Drawing for the job (mm, zero at the part's lowest x, y, z). Give positions to 0.01 mm unless a question says otherwise; leave off trailing zeros. Loops run counter-clockwise (first coordinate to the right, second up) from the corner with the lowest first, then second, coordinate; pieces in that order, holes last. Notation, with made-up numbers: (26, 57) - (73, 57) arc R14 ccw to (73, 64) - close; hole circle Ø4 at (56.25, -38.75). An arc over 180 degrees is marked (long way). Return JSON: item names as keys, results as strings. Group by question number.
1) Drill centre lines: probe 1 along Y at (x, z) = (97.5, 2.65); probe 2 along X at (y, z) = (69.5, 3.3); probe 3 along Y at (x, z) = (52.5, 9.5). Where is each one in solid material? Low to high. Write a range as from..to.
2) Slice it at C-C (z = 10). List the corners of the cut face in (x, y).
3) Drop flat-ended pins along their axis: pin 1 (6.5 mm diameter, centred on x = 105.5, z = 3, fed in from -Y); pin 2 (2.5 mm diameter, centred on x = 27.5, y = 3, fed in from +Z); pin 3 (0.8 mm diameter, centred on y = 64.5, z = 3, fed in from +X). Give the stop position or say it passes through.
4) Slice it at A-A (y = 36). List the corners of the cut face in (x, z).
5) Slice it at B-B (x = 49). List the corners of the cut face in (y, z).
6) Mould opens along X. For the marked faces 1, 2, 3 and 4 say: released by +X, released by -X, zero draft, split by the parting line, or undercut.
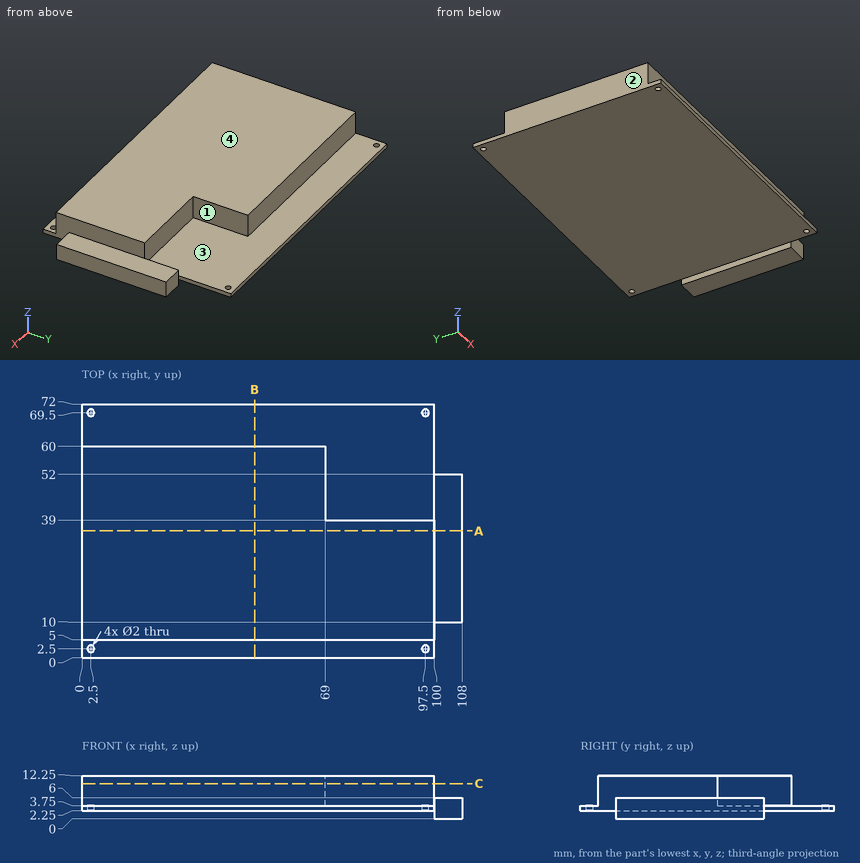
Results:
{
 "1": {"probe 1": "0..1.5, 3.5..68.5, 70.5..72", "probe 2": "0..1.5, 3.5..96.5, 98.5..100", "probe 3": "5..60"},
 "2": {"outline": "(0, 5) - (100, 5) - (100, 39) - (69, 39) - (69, 60) - (0, 60) - close"},
 "3": {"pin 1": "y = 10", "pin 2": "z = 3.75", "pin 3": "x = 100"},
 "4": {"outline": "(0, 2.25) - (100, 2.25) - (100, 0) - (108, 0) - (108, 6) - (100, 6) - (100, 12.25) - (0, 12.25) - close"},
 "5": {"outline": "(0, 2.25) - (72, 2.25) - (72, 3.75) - (60, 3.75) - (60, 12.25) - (5, 12.25) - (5, 3.75) - (0, 3.75) - close"},
 "6": {"face 1": "undercut", "face 2": "released by -X", "face 3": "undercut", "face 4": "zero draft"}
}
